Can you work these out from the model? Positions are in its coordinate system, mm. Face numbers are marked on the shaded views. Round coordinates to 2 decimals unless told otherwise and drop trailing zeros. Write each loop counter-clockwise with the first axis right and the second up, starting at its lowest first coordinate (ties: lowest second). Pieces come first, ordered by that corner, then holes. Notation, with made-up numbers: (81, 22.5) -> (92, 22.5) arc R23 ccw to (92, 55.5) -> close; hole circle Ø2 at (37, 47.25). An arc over 180 degrees is marked (long way). Use CSV: the item, a comma, the result in double quotes.
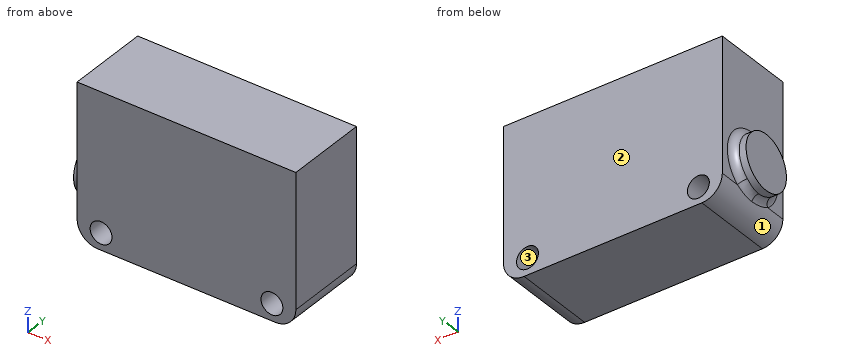
```python
from build123d import *

# Parameters (mm, degrees)
SKETCH_1_R      = 1.6
EXTRUDE_1_DEPTH = 6
SKETCH_2_R      = 4
EXTRUDE_2_DEPTH = 2
FILLET_1_R      = 1


with BuildPart() as part:
    # 草图1 → 凸台-拉伸1 (new, symmetric)
    with BuildSketch(Plane(origin=(0, 0, 0), x_dir=(1, 0, 0), z_dir=(0, 1, 0))):
        with BuildLine():
            Line((-16, -11.25), (16, -11.25))
            Line((16, -11.25), (16, 8.25))
            ThreePointArc((16, 8.25), (15.121320344, 10.371320344), (13, 11.25))
            Line((13, 11.25), (-13, 11.25))
            ThreePointArc((-13, 11.25), (-15.121320344, 10.371320344), (-16, 8.25))
            Line((-16, 8.25), (-16, -11.25))
        make_face()
        with Locations(Location((12.5, 8.7890625, 0), (0, 0, 270))):
            Circle(SKETCH_1_R, mode=Mode.SUBTRACT)
        with Locations(Location((-12.5, 8.7890625, 0), (0, 0, 90))):
            Circle(SKETCH_1_R, mode=Mode.SUBTRACT)
    extrude(amount=EXTRUDE_1_DEPTH, both=True)

    # 草图2 → 凸台-拉伸2 (add)
    with BuildSketch(Plane.ZY.offset(16)):
        with Locations(Location((-4.25, 0, 0), (0, 0, 180))):
            Circle(SKETCH_2_R)
    extrude(amount=EXTRUDE_2_DEPTH)

    # 圆角1
    fillet_1_edges = [part.edges().sort_by_distance(p)[0] for p in [
        (-16, 0, -0.25),
    ]]
    fillet(fillet_1_edges, radius=FILLET_1_R)


solid = part.part
```
Q1. Please list where these lines run through material, in increasing order: probe 1 along X at (y, z) = (0.25, -7.5); probe 2 along Z at (x, y) = (-12.5, -1.75); probe 3 along X at (y, z) = (3.5, -8.25).
Resolved:
probe 1,"x = -18 to -13.45, -11.55 to 11.55, 13.45 to 16"
probe 2,"z = -11.25 to -10.39, -7.19 to 11.25"
probe 3,"x = -16 to -14.01, -10.99 to 10.99, 14.01 to 16"
Q2. Will this pin go through, and if not, where does the flat tip stop? P1, Ø3.5, axis at y = 0.5, z = 4, coming from the -X side.
Resolved:
P1,"stops at x = -16"
Q3. Suppose I cut it at A-A (x = 12.5). Write out the boundary of the cut face in (y, z).
Resolved:
outline,"(-6, -11.25) -> (6, -11.25) -> (6, -10.39) -> (-6, -10.39) -> close; (-6, -7.19) -> (6, -7.19) -> (6, 11.25) -> (-6, 11.25) -> close"
Q4. Suppose I cut it at B-B (z = -4.25). Write out the boundary of the cut face in (x, y).
Resolved:
outline,"(-18, -4) -> (-17, -4) arc R1 cw to (-16, -5) -> (-16, -6) -> (16, -6) -> (16, 6) -> (-16, 6) -> (-16, 5) arc R1 cw to (-17, 4) -> (-18, 4) -> close"
Q5. Suppose I cut it at C-C (z = 2.5). Write out the boundary of the cut face in (x, y).
Resolved:
outline,"(-16, -6) -> (16, -6) -> (16, 6) -> (-16, 6) -> close"
Q6. If we mould it in two halves opening along Z, with no side actions, what happens to the marked faces 1, 2 and 3? For each: released by +Z, released by -Z, zero draft, split by the parting line, or undercut.
Resolved:
face 1,"released by -Z"
face 2,"zero draft"
face 3,"undercut"
